Part model, mm, in its own coordinate system. A direction names the side the tool comes from. Coordinates: 2 decimals unless noted, no trailing zeros. Order: outer loops, then holes, each group sorted by start corner. A loop starts at its lowest first (then second) coordinate and runs counter-clockwise, first axis right, second up.
from build123d import *

# Parameters (mm, degrees)
SM_START                           = -40.6
SM_BASE_FLANGE_1_OUTLINE_W         = 2
SM_BASE_FLANGE_1_OUTLINE_H         = 90
SM_BASE_FLANGE_1_DEPTH             = 81.2
SKETCH_6_R                         = 17.5
CUT_EXTRUDE_1_DEPTH                = 10
F_7_1_7_1_DIAMETER_HOLE1_D         = 7.1
SM_EDGE_FLANGE_1_DEPTH             = 90
SM_EDGE_FLANGE_1_BEND_DEPTH        = 90
SM_EDGE_FLANGE_2_STRIP_W           = 12.8
SM_EDGE_FLANGE_2_STRIP_H           = 2
SM_EDGE_FLANGE_2_STRIP_CUT_DEPTH   = 90
SM_EDGE_FLANGE_2_STRIP_2_W         = 12.8
SM_EDGE_FLANGE_2_STRIP_2_H         = 2
SM_EDGE_FLANGE_2_STRIP_CUT_2_DEPTH = 90
SM_EDGE_FLANGE_2_DEPTH             = 90
SM_EDGE_FLANGE_2_BEND_DEPTH        = 90
CUT_EXTRUDE1_DEPTH                 = 118.273185341
FILLET_2_R                         = 10
F_10_5_10_5_DIAMETER_HOLE1_D       = 10.5


# Read off the part's stored shape, not the designer's step: Базовая кромка1
# Sheet-metal steps are written as plain solids
with BuildPart() as part:
    # Базовая кромка1 outline → Базовая кромка1 (new body)
    with BuildSketch(Plane(origin=(0, 0, 0), x_dir=(0, 0, -1), z_dir=(1, 0, 0)).offset(SM_START)):
        with Locations((1, 45)):
            Rectangle(SM_BASE_FLANGE_1_OUTLINE_W, SM_BASE_FLANGE_1_OUTLINE_H)
    extrude(amount=SM_BASE_FLANGE_1_DEPTH)

    # Эскиз6 → Вырез-Вытянуть1 (cut)
    with BuildSketch(Plane.XY):
        with Locations((0, 35)):
            Circle(SKETCH_6_R)
    extrude(amount=-CUT_EXTRUDE_1_DEPTH, mode=Mode.SUBTRACT)

    # Ø7.1 (7.1) Diameter Hole1 (through all)
    with Locations(Plane.XY):
        with Locations((-33.234018716, 83.234018716), (33.234018716, 83.234018716), (33.234018716, 16.765981284), (-33.234018716, 16.765981284)):
            Hole(F_7_1_7_1_DIAMETER_HOLE1_D / 2)

    # Ребро-кромка1 section (across the edge) → Ребро-кромка1 (add)
    with BuildSketch(Plane(origin=(43, 0, 0), x_dir=(-1, 0, 0), z_dir=(0, 1, 0))):
        with BuildLine():
            Line((-2, 2.4), (-2, 18))
            Line((-2, 18), (0, 18))
            Line((0, 18), (0, 2.4))
            ThreePointArc((0, 2.4), (0.702943725, 0.702943725), (2.4, 0))
            Line((2.4, 0), (2.4, -2))
            ThreePointArc((2.4, -2), (-0.711269837, -0.711269837), (-2, 2.4))
        make_face()
    extrude(amount=SM_EDGE_FLANGE_1_DEPTH)

    # Ребро-кромка1 section 2 (across the edge) → Ребро-кромка1 bend (add)
    with BuildSketch(Plane(origin=(-43, 90, 0), x_dir=(1, 0, 0), z_dir=(0, -1, 0))):
        with BuildLine():
            Line((-2, 2.4), (-2, 18))
            Line((-2, 18), (0, 18))
            Line((0, 18), (0, 2.4))
            ThreePointArc((0, 2.4), (0.702943725, 0.702943725), (2.4, 0))
            Line((2.4, 0), (2.4, -2))
            ThreePointArc((2.4, -2), (-0.711269837, -0.711269837), (-2, 2.4))
        make_face()
    extrude(amount=SM_EDGE_FLANGE_1_BEND_DEPTH)

    # Ребро-кромка2 strip (across the edge) → Ребро-кромка2 strip cut (cut)
    with BuildSketch(Plane(origin=(45, 90, 18), x_dir=(0, 0, -1), z_dir=(0, -1, 0))):
        with Locations((-2, -1)):
            Rectangle(SM_EDGE_FLANGE_2_STRIP_W, SM_EDGE_FLANGE_2_STRIP_H)
    extrude(amount=SM_EDGE_FLANGE_2_STRIP_CUT_DEPTH, mode=Mode.SUBTRACT)

    # Ребро-кромка2 strip 2 (across the edge) → Ребро-кромка2 strip cut 2 (cut)
    with BuildSketch(Plane(origin=(-45, 0, 18), x_dir=(0, 0, -1), z_dir=(0, 1, 0))):
        with Locations((-2, -1)):
            Rectangle(SM_EDGE_FLANGE_2_STRIP_2_W, SM_EDGE_FLANGE_2_STRIP_2_H)
    extrude(amount=SM_EDGE_FLANGE_2_STRIP_CUT_2_DEPTH, mode=Mode.SUBTRACT)

    # Ребро-кромка2 section (across the edge) → Ребро-кромка2 (add)
    with BuildSketch(Plane(origin=(45, 90, 18), x_dir=(0, 0, -1), z_dir=(0, -1, 0))):
        with BuildLine():
            Line((0, 2.4), (0, 28))
            Line((0, 28), (2, 28))
            Line((2, 28), (2, 2.4))
            ThreePointArc((2, 2.4), (2.702943725, 0.702943725), (4.4, 0))
            Line((4.4, 0), (4.4, -2))
            ThreePointArc((4.4, -2), (1.288730163, -0.711269837), (0, 2.4))
        make_face()
    extrude(amount=SM_EDGE_FLANGE_2_DEPTH)

    # Ребро-кромка2 section 2 (across the edge) → Ребро-кромка2 bend (add)
    with BuildSketch(Plane(origin=(-45, 0, 18), x_dir=(0, 0, -1), z_dir=(0, 1, 0))):
        with BuildLine():
            Line((0, 2.4), (0, 28))
            Line((0, 28), (2, 28))
            Line((2, 28), (2, 2.4))
            ThreePointArc((2, 2.4), (2.702943725, 0.702943725), (4.4, 0))
            Line((4.4, 0), (4.4, -2))
            ThreePointArc((4.4, -2), (1.288730163, -0.711269837), (0, 2.4))
        make_face()
    extrude(amount=SM_EDGE_FLANGE_2_BEND_DEPTH)

    # Sketch4 → Cut-Extrude1 (cut, through all)
    with BuildSketch(Plane(origin=(0, 0, 16), x_dir=(-1, 0, 0), z_dir=(0, 0, -1))):
        Polygon((-73, 90), (-58, 90), (-73, 45), align=None)
        Polygon((-73, 25), (-58, 0), (-73, 0), align=None)
        Polygon((73, 0), (73, 25), (58, 0), align=None)
        Polygon((58, 90), (73, 45), (73, 90), align=None)
    extrude(amount=-CUT_EXTRUDE1_DEPTH, mode=Mode.SUBTRACT)

    # Скругление2
    fillet_2_edges = [part.edges().sort_by_distance(p)[0] for p in [
        (-58, 90, 17),
        (-73, 45, 17),
        (-58, 0, 17),
        (-73, 25, 17),
        (73, 25, 17),
        (58, 0, 17),
        (73, 45, 17),
        (58, 90, 17),
    ]]
    fillet(fillet_2_edges, radius=FILLET_2_R)

    # Ø10.5 (10.5) Diameter Hole1 (through all)
    with Locations(Plane(origin=(0, 0, -2), x_dir=(-1, 0, 0), z_dir=(0, 0, -1))):
        with Locations((-58.5, 35), (58.5, 35)):
            Hole(F_10_5_10_5_DIAMETER_HOLE1_D / 2)


solid = part.part
Q1. Cut at B-B on z = 12. Write the cut outline in (x, y).
Results list:
outline: (-45, 0) - (-43, 0) - (-43, 90) - (-45, 90) - close; (43, 0) - (45, 0) - (45, 90) - (43, 90) - close
Q2. Which spindle directions (+Z, -Z, +X, -X, +Y, -Y) get a long thin tool onto all of the face, cutting with end or side? Do faces 1 (the face through (-44.255, 44.37, 16.677)), 2 (the face through (-58, 44, 16)), 3 (the face through (58, 46, 16)). Say none if no direction does.
Results list:
face 1: +Z, +Y, -Y
face 2: -Z, -X, +Y, -Y
face 3: -Z, +X, +Y, -Y
Q3. Pin check, flat tips, straight feed: pin 1 Ø3 at (x, y) = (-29, 24.5) entering from +Z; pin 2 Ø5 at (y, z) = (24, 12.5) entering from -X; pin 3 Ø20.5 at (x, y) = (66, 24) entering from -Z. Stop position of each tip, or through.
Results list:
pin 1: stops at z = 0
pin 2: stops at x = -45.45
pin 3: stops at z = 16
Q4. Wall check: line 1 along X through (y, z) = (13, 9.5); line 2 along Z through (x, y) = (51.5, 78); line 3 along Z through (x, y) = (19.5, 25). Give the ranges that are in metal, low to high.
Results list:
line 1: x = -45 to -43, 43 to 45
line 2: z = 16 to 18
line 3: z = -2 to 0
Q5. Cut at D-D on y = 60.5. Write the cut outline in (x, z).
Results list:
outline: (-67.83, 16) - (-47.4, 16) arc R2.4 cw to (-45, 13.6) - (-45, 2.4) arc R4.4 ccw to (-40.6, -2) - (40.6, -2) arc R4.4 ccw to (45, 2.4) - (45, 13.6) arc R2.4 cw to (47.4, 16) - (67.83, 16) - (67.83, 18) - (47.4, 18) arc R4.4 ccw to (43, 13.6) - (43, 2.4) arc R2.4 cw to (40.6, 0) - (-40.6, 0) arc R2.4 cw to (-43, 2.4) - (-43, 13.6) arc R4.4 ccw to (-47.4, 18) - (-67.83, 18) - close
Q6. Cut at C-C on y = 35. Count the separate pieces of the cut face and the enclosed holes in it, and give its area (3 significant figures).
Results list:
separate pieces: 4
enclosed holes: 0
area: 240 mm2
Q7. Cut at A-A on x = 0. Write the cut outline in (y, z), and give its area (3 significant figures).
Results list:
outline: (0, -2) - (17.5, -2) - (17.5, 0) - (0, 0) - close; (52.5, -2) - (90, -2) - (90, 0) - (52.5, 0) - close
area: 110 mm2
Q8. Mould opens along X. For faces 4 (the face through (-0.2, 0, -0.2)), 5 (the face through (-56.71, 88.06, 17.01)), 6 (the face through (33.696, 86.754, -1.014)) say: pulls with the +X half, pulls with the -X half, needs draft (parallel to the pull), parting line crosses it, or undercut.
Results list:
face 4: needs draft
face 5: pulls with the -X half
face 6: undercut
